Geometry: see drawing. Coordinates: mm, zero at the bounding-box minimum. Round coordinates to 2 decimals unless told otherwise and drop trailing zeros. Order: outer loops, then holes, each group sorted by start corner. A loop starts at its lowest first (then second) coordinate and runs counter-clockwise, first axis right, second up. Notation, with made-up numbers: (8, -10) -> (24, -10) arc R20 cw to (24, 5) -> close; hole circle Ø2 at (41.5, 33.25). An arc over 180 degrees is marked (long way). Answer as CSV lines item,"result". Start each with the question number.
(1) Section query A-A (y = 11). Output: boundary loops of the cut face in (x, z), plus the area to 3 significant figures.
(2) Contact query for flat-ended pins moving along their axis: P1, Ø24, axis at x = 37.5, z = 16.5, coming from the -Y side; P2, Ø3, axis at x = 38.5, y = 15, coming from the -Z side. Output: stop coordinate, or through.
(3) Line query: line 1 along Z through (x, y) = (20, 18). Output: solid intervals per line, ascending. Write a range as from..to.
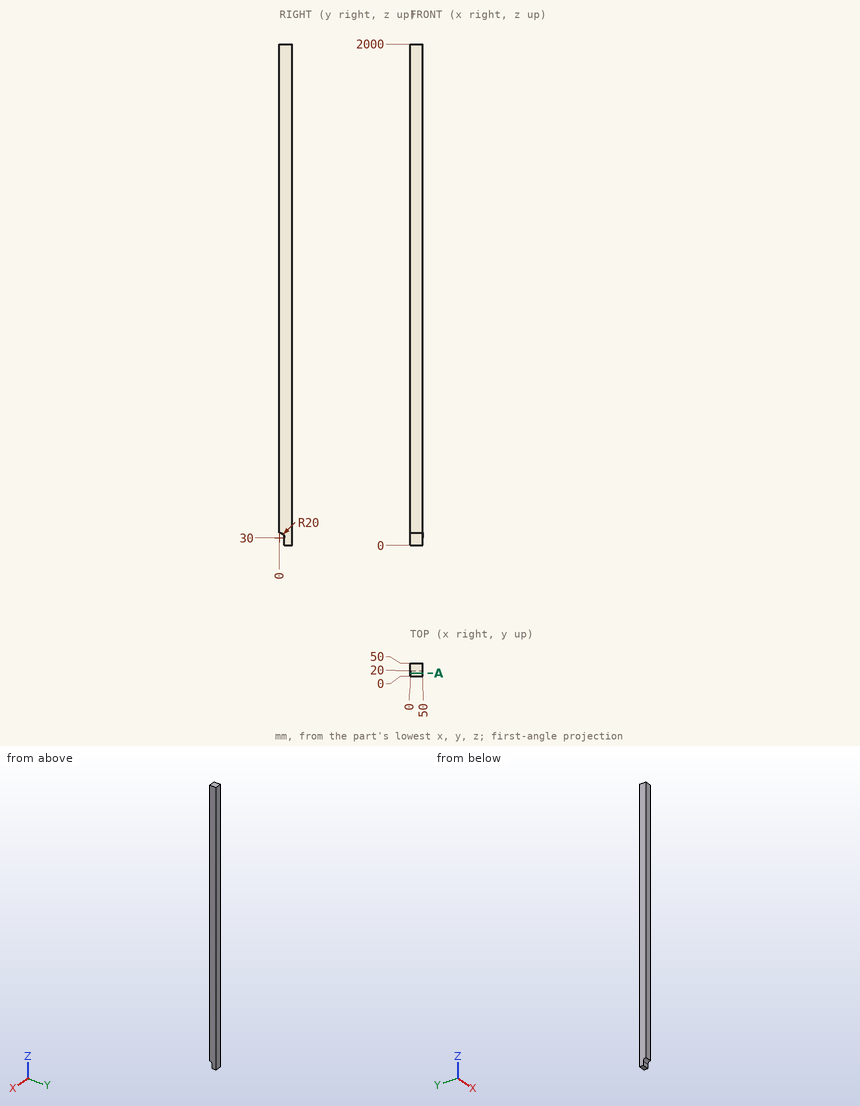
Answer block:
1,outline,"(0, 46.7) -> (50, 46.7) -> (50, 2000) -> (0, 2000) -> close"
1,area,"97,700 mm2"
2,P1,"y = 20"
2,P2,"z = 41.3"
3,line 1,"38.72..2000"
